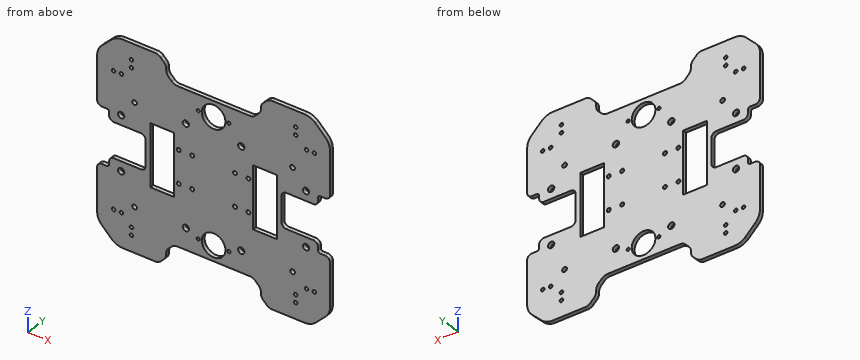
```python
from build123d import *

# Parameters (mm, degrees)
SKETCH2_W                                     = 30
SKETCH2_H                                     = 80
BASE_DEPTH                                    = 5
SKETCH3_R                                     = 4
ENCODER_MOUNTING_ORIGINAL_BR_DEPTH            = 5
ENCODER_MOUNTING_SYM_XL_COPY_1_SKETCH_R       = 4
ENCODER_MOUNTING_SYM_XL_COPY_1_DEPTH          = 5
SKETCH4_R                                     = 2.5
WHEEL_GUIDES_MOUNTING_ORIGINAL_XR_DEPTH       = 5
SKETCH6_R                                     = 3
FRAME_MOUNTING_DEPTH                          = 5
SKETCH5_R                                     = 4
SUPPORT_MOTEUR_MOUNTING_INSIDE_ORIGINAL_DEPTH = 5
SKETCH13_R                                    = 15
SKETCH13_R_2                                  = 2
SCROLLERS_MOUNTINGS_DEPTH                     = 5
CHAMFER1_SIZE                                 = 24
FILLET1_R                                     = 20
ESQUISSE1_W                                   = 120
ESQUISSE1_H                                   = 30
ENL_V_MAT_EXTRU_1_DEPTH                       = 197.675494152
CHANFREIN1_SIZE                               = 10
CONG_1_R                                      = 10
CHANFREIN2_SIZE                               = 10
CONG_2_R                                      = 10
ESQUISSE2_R                                   = 2.25
ENL_V_MAT_EXTRU_2_DEPTH                       = 197.675494152
ESQUISSE3_R                                   = 2.25
ENL_V_MAT_EXTRU_3_DEPTH                       = 197.675494152
ESQUISSE4_R                                   = 2.25
ENL_V_MAT_EXTRU_4_DEPTH                       = 197.675494152
ESQUISSE5_R                                   = 2.25
ENL_V_MAT_EXTRU_5_DEPTH                       = 197.675494152


with BuildPart() as part:
    # Sketch2 → Base (new body)
    with BuildSketch(Plane(origin=(0, 0, 0), x_dir=(1, 0, 0), z_dir=(0, 1, 0))):
        with BuildLine():
            Line((-147.5, -130), (147.5, -130))
            Line((147.5, -130), (147.5, -41.75500004))
            ThreePointArc((147.5, -41.75500004), (145.742640687, -37.512359353), (141.5, -35.75500004))
            Line((141.5, -35.75500004), (135.3, -35.75500004))
            ThreePointArc((135.3, -35.75500004), (133.178679656, -34.876320383), (132.3, -32.75500004))
            Line((132.3, -32.75500004), (132.3, -28.530608474))
            ThreePointArc((132.3, -28.530608474), (130.542640675, -24.287967759), (126.29999996, -22.530608435))
            Line((126.29999996, -22.530608435), (92.090541187, -22.530608435))
            ThreePointArc((92.090541187, -22.530608435), (87.8479005, -20.773249122), (86.090541187, -16.530608435))
            Line((86.090541187, -16.530608435), (86.090541187, 16.530608435))
            ThreePointArc((86.090541187, 16.530608435), (87.8479005, 20.773249122), (92.090541187, 22.530608435))
            Line((92.090541187, 22.530608435), (126.29999996, 22.530608435))
            ThreePointArc((126.29999996, 22.530608435), (130.542640675, 24.287967759), (132.3, 28.530608474))
            Line((132.3, 28.530608474), (132.3, 32.75500004))
            ThreePointArc((132.3, 32.75500004), (133.178679656, 34.876320383), (135.3, 35.75500004))
            Line((135.3, 35.75500004), (141.5, 35.75500004))
            ThreePointArc((141.5, 35.75500004), (145.742640687, 37.512359353), (147.5, 41.75500004))
            Line((147.5, 41.75500004), (147.5, 130))
            Line((147.5, 130), (-147.5, 130))
            Line((-147.5, 130), (-147.5, 41.75500004))
            ThreePointArc((-147.5, 41.75500004), (-145.742640687, 37.512359353), (-141.5, 35.75500004))
            Line((-141.5, 35.75500004), (-135.3, 35.75500004))
            ThreePointArc((-135.3, 35.75500004), (-133.178679656, 34.876320383), (-132.3, 32.75500004))
            Line((-132.3, 32.75500004), (-132.3, 28.530608474))
            ThreePointArc((-132.3, 28.530608474), (-130.542640675, 24.287967759), (-126.29999996, 22.530608435))
            Line((-126.29999996, 22.530608435), (-92.090541187, 22.530608435))
            ThreePointArc((-92.090541187, 22.530608435), (-87.8479005, 20.773249122), (-86.090541187, 16.530608435))
            Line((-86.090541187, 16.530608435), (-86.090541187, -16.530608435))
            ThreePointArc((-86.090541187, -16.530608435), (-87.8479005, -20.773249122), (-92.090541187, -22.530608435))
            Line((-92.090541187, -22.530608435), (-126.29999996, -22.530608435))
            ThreePointArc((-126.29999996, -22.530608435), (-130.542640675, -24.287967759), (-132.3, -28.530608474))
            Line((-132.3, -28.530608474), (-132.3, -32.75500004))
            ThreePointArc((-132.3, -32.75500004), (-133.178679656, -34.876320383), (-135.3, -35.75500004))
            Line((-135.3, -35.75500004), (-141.5, -35.75500004))
            ThreePointArc((-141.5, -35.75500004), (-145.742640687, -37.512359353), (-147.5, -41.75500004))
            Line((-147.5, -41.75500004), (-147.5, -130))
        make_face()
        with Locations((65.090541187, 0)):
            Rectangle(SKETCH2_W, SKETCH2_H, mode=Mode.SUBTRACT)
        with Locations((-65.090541187, 0)):
            Rectangle(SKETCH2_W, SKETCH2_H, mode=Mode.SUBTRACT)
    extrude(amount=BASE_DEPTH)

    # Sketch3 → Encoder Mounting-Original_BR (cut)
    with BuildSketch(Plane(origin=(0, 5, 0), x_dir=(1, 0, 0), z_dir=(0, 1, 0))):
        with Locations(Location((117.1, -35.000608435, 0), (0, 0, 270))):
            Circle(SKETCH3_R)
    encoder_mounting_original_br = extrude(amount=-ENCODER_MOUNTING_ORIGINAL_BR_DEPTH, mode=Mode.SUBTRACT)

    # Encoder Mounting-Sym_FR: Encoder Mounting-Original_BR across plane
    add(encoder_mounting_original_br.mirror(Plane(origin=(0, 0, 0), x_dir=(1, 0, 0), z_dir=(0, 0, -1))), mode=Mode.SUBTRACT)

    # Encoder Mounting-Sym_xL: Encoder Mounting-Original_BR across plane
    add(encoder_mounting_original_br.mirror(Plane(origin=(0, 0, 0), x_dir=(0, 0, 1), z_dir=(1, 0, 0))), mode=Mode.SUBTRACT)

    # Encoder Mounting-Sym_xL copy 1 sketch → Encoder Mounting-Sym_xL copy 1 (cut)
    with BuildSketch(Plane(origin=(0, 5, 0), x_dir=(-1, 0, 0), z_dir=(0, 1, 0))):
        with Locations(Location((117.1, -35.000608435, 0), (0, 0, 270))):
            Circle(ENCODER_MOUNTING_SYM_XL_COPY_1_SKETCH_R)
    extrude(amount=-ENCODER_MOUNTING_SYM_XL_COPY_1_DEPTH, mode=Mode.SUBTRACT)

    # Sketch4 → Wheel Guides Mounting-Original_xR (cut)
    with BuildSketch(Plane(origin=(0, 5, 0), x_dir=(1, 0, 0), z_dir=(0, 1, 0))):
        with Locations(Location((44.090541187, -21, 0), (0, 0, 270))):
            Circle(SKETCH4_R)
        with Locations(Location((27.090541187, -21, 0), (0, 0, 270))):
            Circle(SKETCH4_R)
        with Locations(Location((27.090541187, 21, 0), (0, 0, 270))):
            Circle(SKETCH4_R)
        with Locations(Location((44.090541187, 21, 0), (0, 0, 270))):
            Circle(SKETCH4_R)
    wheel_guides_mounting_original_xr = extrude(amount=-WHEEL_GUIDES_MOUNTING_ORIGINAL_XR_DEPTH, mode=Mode.SUBTRACT)

    # Wheel Guides Mounting-Sym_xL: Wheel Guides Mounting-Original_xR across plane
    add(wheel_guides_mounting_original_xr.mirror(Plane(origin=(0, 0, 0), x_dir=(0, 0, 1), z_dir=(1, 0, 0))), mode=Mode.SUBTRACT)

    # Sketch6 → Frame Mounting (cut)
    with BuildSketch(Plane(origin=(0, 5, 0), x_dir=(1, 0, 0), z_dir=(0, 1, 0))):
        with Locations(Location((100.090541187, -57.469391565, 0), (0, 0, 270))):
            Circle(SKETCH6_R)
        with Locations(Location((-100.090541187, -57.469391565, 0), (0, 0, 270))):
            Circle(SKETCH6_R)
        with Locations(Location((100.090541187, 72.530608435, 0), (0, 0, 270))):
            Circle(SKETCH6_R)
        with Locations(Location((-100.090541187, 72.530608435, 0), (0, 0, 270))):
            Circle(SKETCH6_R)
    extrude(amount=-FRAME_MOUNTING_DEPTH, mode=Mode.SUBTRACT)

    # Sketch5 → Support Moteur Mounting Inside-Original (cut)
    with BuildSketch(Plane(origin=(0, 5, 0), x_dir=(1, 0, 0), z_dir=(0, 1, 0))):
        with Locations(Location((35.090541187, -57.469391565, 0), (0, 0, 270))):
            Circle(SKETCH5_R)
        with Locations(Location((35.090541187, 72.530608435, 0), (0, 0, 270))):
            Circle(SKETCH5_R)
    support_moteur_mounting_inside_original = extrude(amount=-SUPPORT_MOTEUR_MOUNTING_INSIDE_ORIGINAL_DEPTH, mode=Mode.SUBTRACT)

    # Support Moteur Mounting Inside-Sym_xL: Support Moteur Mounting Inside-Original across plane
    add(support_moteur_mounting_inside_original.mirror(Plane(origin=(0, 0, 0), x_dir=(0, 0, 1), z_dir=(1, 0, 0))), mode=Mode.SUBTRACT)

    # Sketch13 → Scrollers Mountings (cut)
    with BuildSketch(Plane(origin=(0, 5, 0), x_dir=(1, 0, 0), z_dir=(0, 1, 0))):
        with Locations(Location((0, -80, 0), (0, 0, 270))):
            Circle(SKETCH13_R)
        with Locations(Location((19.5, -80, 0), (0, 0, 270))):
            Circle(SKETCH13_R_2)
        with Locations(Location((-19.5, -80, 0), (0, 0, 270))):
            Circle(SKETCH13_R_2)
        with Locations(Location((0, 80, 0), (0, 0, 270))):
            Circle(SKETCH13_R)
        with Locations(Location((19.5, 80, 0), (0, 0, 270))):
            Circle(SKETCH13_R_2)
        with Locations(Location((-19.5, 80, 0), (0, 0, 270))):
            Circle(SKETCH13_R_2)
    extrude(amount=-SCROLLERS_MOUNTINGS_DEPTH, mode=Mode.SUBTRACT)

    # Chamfer1
    chamfer1_edges = [part.edges().sort_by_distance(p)[0] for p in [
        (147.5, 2.5, 130),
        (-147.5, 2.5, 130),
        (-147.5, 2.5, -130),
        (147.5, 2.5, -130),
    ]]
    chamfer(chamfer1_edges, length=CHAMFER1_SIZE)

    # Fillet1
    fillet1_edges = [part.edges().sort_by_distance(p)[0] for p in [
        (-123.5, 2.5, -130),
        (123.5, 2.5, -130),
        (147.5, 2.5, -106),
        (-147.5, 2.5, -106),
        (147.5, 2.5, 106),
        (-123.5, 2.5, 130),
        (123.5, 2.5, 130),
        (-147.5, 2.5, 106),
    ]]
    fillet(fillet1_edges, radius=FILLET1_R)

    # Esquisse1 → Enl_v. mat.-Extru.1 (cut, through all)
    with BuildSketch(Plane(origin=(0, 5, 0), x_dir=(1, 0, 0), z_dir=(0, 1, 0))):
        with Locations((0, 115)):
            Rectangle(ESQUISSE1_W, ESQUISSE1_H)
    enl_v_mat_extru_1 = extrude(amount=-ENL_V_MAT_EXTRU_1_DEPTH, mode=Mode.SUBTRACT)

    # Chanfrein1
    chanfrein1_edges = [part.edges().sort_by_distance(p)[0] for p in [
        (60, 2.5, -130),
        (60, 2.5, -100),
        (-60, 2.5, -100),
        (-60, 2.5, -130),
    ]]
    chamfer(chanfrein1_edges, length=CHANFREIN1_SIZE)

    # Cong_1
    cong_1_edges = [part.edges().sort_by_distance(p)[0] for p in [
        (50, 2.5, -100),
        (-50, 2.5, -100),
        (-60, 2.5, -120),
        (-60, 2.5, -110),
        (60, 2.5, -120),
        (60, 2.5, -110),
        (-70, 2.5, -130),
        (70, 2.5, -130),
    ]]
    fillet(cong_1_edges, radius=CONG_1_R)

    # Sym_trie1: Enl_v. mat.-Extru.1 across plane
    add(enl_v_mat_extru_1.mirror(Plane.XY), mode=Mode.SUBTRACT)

    # Chanfrein2
    chanfrein2_edges = [part.edges().sort_by_distance(p)[0] for p in [
        (60, 2.5, 100),
        (60, 2.5, 130),
        (-60, 2.5, 130),
        (-60, 2.5, 100),
    ]]
    chamfer(chanfrein2_edges, length=CHANFREIN2_SIZE)

    # Cong_2
    cong_2_edges = [part.edges().sort_by_distance(p)[0] for p in [
        (-70, 2.5, 130),
        (-60, 2.5, 110),
        (-60, 2.5, 120),
        (50, 2.5, 100),
        (-50, 2.5, 100),
        (60, 2.5, 120),
        (60, 2.5, 110),
        (70, 2.5, 130),
    ]]
    fillet(cong_2_edges, radius=CONG_2_R)

    # Esquisse2 → Enl_v. mat.-Extru.2 (cut, through all)
    with BuildSketch(Plane(origin=(0, 5, 0), x_dir=(1, 0, 0), z_dir=(0, 1, 0))):
        with Locations(Location((117.75, 86.5, 0), (0, 0, 270))):
            Circle(ESQUISSE2_R)
        with Locations(Location((127.75, 86.5, 0), (0, 0, 270))):
            Circle(ESQUISSE2_R)
    enl_v_mat_extru_2 = extrude(amount=-ENL_V_MAT_EXTRU_2_DEPTH, mode=Mode.SUBTRACT)

    # Esquisse3 → Enl_v. mat.-Extru.3 (cut, through all)
    with BuildSketch(Plane(origin=(0, 5, 0), x_dir=(1, 0, 0), z_dir=(0, 1, 0))):
        with Locations(Location((104, 109.45, 0), (0, 0, 270))):
            Circle(ESQUISSE3_R)
        with Locations(Location((104, 99.45, 0), (0, 0, 270))):
            Circle(ESQUISSE3_R)
    enl_v_mat_extru_3 = extrude(amount=-ENL_V_MAT_EXTRU_3_DEPTH, mode=Mode.SUBTRACT)

    # Esquisse4 → Enl_v. mat.-Extru.4 (cut, through all)
    with BuildSketch(Plane(origin=(0, 5, 0), x_dir=(1, 0, 0), z_dir=(0, 1, 0))):
        with Locations(Location((-126.75, 86.5, 0), (0, 0, 270))):
            Circle(ESQUISSE4_R)
        with Locations(Location((-116.75, 86.5, 0), (0, 0, 270))):
            Circle(ESQUISSE4_R)
    enl_v_mat_extru_4 = extrude(amount=-ENL_V_MAT_EXTRU_4_DEPTH, mode=Mode.SUBTRACT)

    # Esquisse5 → Enl_v. mat.-Extru.5 (cut, through all)
    with BuildSketch(Plane(origin=(0, 5, 0), x_dir=(1, 0, 0), z_dir=(0, 1, 0))):
        with Locations(Location((-104, -99.25, 0), (0, 0, 270))):
            Circle(ESQUISSE5_R)
        with Locations(Location((-104, -109.25, 0), (0, 0, 270))):
            Circle(ESQUISSE5_R)
    extrude(amount=-ENL_V_MAT_EXTRU_5_DEPTH, mode=Mode.SUBTRACT)

    # Sym_trie2: Enl_v. mat.-Extru.2, Enl_v. mat.-Extru.3 across plane
    add(enl_v_mat_extru_2.mirror(Plane.XY), mode=Mode.SUBTRACT)
    add(enl_v_mat_extru_3.mirror(Plane.XY), mode=Mode.SUBTRACT)

    # Sym_trie3: Enl_v. mat.-Extru.3 across plane
    add(enl_v_mat_extru_3.mirror(Plane(origin=(0, 0, 0), x_dir=(0, 0, 1), z_dir=(1, 0, 0))), mode=Mode.SUBTRACT)

    # Sym_trie4: Enl_v. mat.-Extru.4 across plane
    add(enl_v_mat_extru_4.mirror(Plane.XY), mode=Mode.SUBTRACT)


solid = part.part
```
Work out the finished part from the listing and answer in its coordinate system (mm). Give positions to 0.01 mm unless a question says otherwise; leave off trailing zeros. Order: outer loops, then holes, each group sorted by start corner. A loop starts at its lowest first (then second) coordinate and runs counter-clockwise, first axis right, second up.
1. Each of these flat-tipped pins is pushed along its axis until it touches: P1, Ø1, axis at y = 0.5, z = -4.5, coming from the -X side; P2, Ø1.5, axis at x = 73.5, y = 3, coming from the -Z side; P3, Ø1.9, axis at y = 3, z = 115, coming from the -X side; P4, Ø0.5, axis at y = 3, z = -115.5, coming from the -X side. Where does it stop, or does it pass through?
Result sheet:
P1: stops at x = -86.09
P2: stops at z = -130
P3: stops at x = -139.45
P4: stops at x = -138.25
2. Section B-B, the plane y = 1.75 is taken. Give the number of separate pieces and of enclosed holes in the cut face, and give its area (3 significant figures).
Result sheet:
separate pieces: 1
enclosed holes: 44
area: 54,700 mm2
3. Section A-A, the plane z = 12 is taken. Determine the outline of the cut face in (x, y).
Result sheet:
outline: (-86.09, 0) - (-80.09, 0) - (-80.09, 5) - (-86.09, 5) - close; (-50.09, 0) - (50.09, 0) - (50.09, 5) - (-50.09, 5) - close; (80.09, 0) - (86.09, 0) - (86.09, 5) - (80.09, 5) - close
4. Straight lines are drawn through the part: L1, parallel to X at y = 4.7, z = 6.5; L2, parallel to X at y = 2.7, z = -99.45; L3, parallel to Z at x = 111.5, y = 1.65. For each, find the intervals that lie inside material, in ascending order.
Result sheet:
L1: x = -86.09 to -80.09, -50.09 to 50.09, 80.09 to 86.09
L2: x = -147.42 to -106.25, -101.75 to 101.75, 106.25 to 147.42
L3: z = -130 to -22.53, 22.53 to 130
